Build history of the part. All positions in model axes, mm. Coordinates: 2 decimals unless noted, no trailing zeros. Order: outer loops, then holes, each group sorted by start corner. A loop starts at its lowest first (then second) coordinate and runs counter-clockwise, first axis right, second up. Notation, with made-up numbers: M -39,68 L -23,68 A18 cw -23,99 Z; hole C 1.5,65 d2. An arc over 180 degrees is marked long. Write item = value, one per line. Start each with the question number.
Q1. Band-saw the part on C-C on x = -243. Write the cut outline in (y, z).
Q2. Band-saw the part on A-A on y = -103. State how many separate pieces and enclosed holes the cut face has, plus the area to 3 significant figures.
Q3. Pin check, flat tips, straight feed: P1, Ø11.5, axis at x = -338.5, z = 202, coming from the -Y side; P2, Ø16, axis at x = 17, y = -20, coming from the +Z side; P3, Ø20, axis at x = -327, y = 292.5, coming from the +Z side. Stop position of each tip, or through.
Q4. Drill centre lines: probe 1 along Y at (x, z) = (17, 211); probe 2 along Z at (x, y) = (-330, 241.9); probe 3 along X at (y, z) = (-29, -30). Where is each one in solid material? Low to high.
Q5. Band-saw the part on B-B on z = -103. Write the cut outline in (x, y).
```python
from build123d import *

# Parameters (mm, degrees)
SKETCH1_W             = 40
SKETCH1_H             = 40
SKETCH1_W_2           = 38
SKETCH1_H_2           = 38
BOSS_EXTRUDE1_DEPTH   = 200
BOSS_EXTRUDE1_2_DEPTH = 200
BOSS_EXTRUDE1_3_DEPTH = 200
BOSS_EXTRUDE1_4_DEPTH = 200
SKETCH2_W             = 700
SKETCH2_H             = 450
SKETCH2_W_2           = 620
SKETCH2_H_2           = 370
BOSS_EXTRUDE2_DEPTH   = 40
SKETCH3_W             = 40
SKETCH3_H             = 40
SKETCH3_W_2           = 38
SKETCH3_H_2           = 38
BOSS_EXTRUDE4_DEPTH   = 100
SKETCH4_R             = 5
CUT_EXTRUDE1_DEPTH    = 465
SKETCH5_W             = 700
SKETCH5_H             = 450
SKETCH5_W_2           = 620
SKETCH5_H_2           = 370
BOSS_EXTRUDE5_DEPTH   = 40
SKETCH6_R             = 5
CUT_EXTRUDE2_DEPTH    = 508
SKETCH7_R             = 38.5
SKETCH7_R_2           = 37.5
BOSS_EXTRUDE6_DEPTH   = 5
SKETCH8_R             = 5
BOSS_EXTRUDE7_DEPTH   = 30


with BuildPart() as part:
    # Sketch1 → Boss-Extrude1 (new body, symmetric)
    with BuildSketch(Plane(origin=(0, 0, 0), x_dir=(1, 0, 0), z_dir=(0, 1, 0))):
        with Locations((-330, 205)):
            Rectangle(SKETCH1_W, SKETCH1_H)
        with Locations((-330, 205)):
            Rectangle(SKETCH1_W_2, SKETCH1_H_2, mode=Mode.SUBTRACT)
    extrude(amount=BOSS_EXTRUDE1_DEPTH, both=True)



with BuildPart() as body_2:
    # Sketch1 → Boss-Extrude1 2 (new body, symmetric)
    with BuildSketch(Plane(origin=(0, 0, 0), x_dir=(1, 0, 0), z_dir=(0, 1, 0))):
        with Locations((330, 205)):
            Rectangle(SKETCH1_W, SKETCH1_H)
        with Locations((330, 205)):
            Rectangle(SKETCH1_W_2, SKETCH1_H_2, mode=Mode.SUBTRACT)
    extrude(amount=BOSS_EXTRUDE1_2_DEPTH, both=True)


with BuildPart() as body_3:
    # Sketch1 → Boss-Extrude1 3 (new body, symmetric)
    with BuildSketch(Plane(origin=(0, 0, 0), x_dir=(1, 0, 0), z_dir=(0, 1, 0))):
        with Locations((330, -205)):
            Rectangle(SKETCH1_W, SKETCH1_H)
        with Locations((330, -205)):
            Rectangle(SKETCH1_W_2, SKETCH1_H_2, mode=Mode.SUBTRACT)
    extrude(amount=BOSS_EXTRUDE1_3_DEPTH, both=True)


with BuildPart() as body_4:
    # Sketch1 → Boss-Extrude1 4 (new body, symmetric)
    with BuildSketch(Plane(origin=(0, 0, 0), x_dir=(1, 0, 0), z_dir=(0, 1, 0))):
        with Locations((-330, -205)):
            Rectangle(SKETCH1_W, SKETCH1_H)
        with Locations((-330, -205)):
            Rectangle(SKETCH1_W_2, SKETCH1_H_2, mode=Mode.SUBTRACT)
    extrude(amount=BOSS_EXTRUDE1_4_DEPTH, both=True)


with BuildPart() as part_1:
    add(part.part)

    add(body_2.part)  # Boss-Extrude2 merges body 2

    add(body_3.part)  # Boss-Extrude2 merges body 3

    add(body_4.part)  # Boss-Extrude2 merges body 4
    # Sketch2 → Boss-Extrude2 (add)
    with BuildSketch(Plane(origin=(0, 200, 0), x_dir=(1, 0, 0), z_dir=(0, 1, 0))):
        Rectangle(SKETCH2_W, SKETCH2_H)
        Rectangle(SKETCH2_W_2, SKETCH2_H_2, mode=Mode.SUBTRACT)
    extrude(amount=BOSS_EXTRUDE2_DEPTH)

    # Sketch3 → Boss-Extrude4 (add)
    with BuildSketch(Plane(origin=(0, 240, 0), x_dir=(1, 0, 0), z_dir=(0, 1, 0))):
        with Locations((-330, 0)):
            Rectangle(SKETCH3_W, SKETCH3_H)
        with Locations((-330, 0)):
            Rectangle(SKETCH3_W_2, SKETCH3_H_2, mode=Mode.SUBTRACT)
        with Locations((330, 0)):
            Rectangle(SKETCH3_W, SKETCH3_H)
        with Locations((330, 0)):
            Rectangle(SKETCH3_W_2, SKETCH3_H_2, mode=Mode.SUBTRACT)
    extrude(amount=BOSS_EXTRUDE4_DEPTH)

    # Sketch4 → Cut-Extrude1 (cut)
    with BuildSketch(Plane.XY.offset(225)):
        with Locations((17, 220)):
            Circle(SKETCH4_R)
    extrude(amount=-CUT_EXTRUDE1_DEPTH, mode=Mode.SUBTRACT)

    # Sketch5 → Boss-Extrude5 (add)
    with BuildSketch(Plane(origin=(0, 0, 0), x_dir=(1, 0, 0), z_dir=(0, 1, 0))):
        Rectangle(SKETCH5_W, SKETCH5_H)
        Rectangle(SKETCH5_W_2, SKETCH5_H_2, mode=Mode.SUBTRACT)
    extrude(amount=-BOSS_EXTRUDE5_DEPTH)

    # Sketch6 → Cut-Extrude2 (cut)
    with BuildSketch(Plane.XY.offset(225)):
        with Locations((17, -20)):
            Circle(SKETCH6_R)
    extrude(amount=-CUT_EXTRUDE2_DEPTH, mode=Mode.SUBTRACT)

    # Sketch7 → Boss-Extrude6 (add)
    with BuildSketch(Plane(origin=(0, 240, 0), x_dir=(1, 0, 0), z_dir=(0, 1, 0))):
        with Locations((-330, 0)):
            Circle(SKETCH7_R)
        with Locations((-330, 0)):
            Circle(SKETCH7_R_2, mode=Mode.SUBTRACT)
        with Locations((330, 0)):
            Circle(SKETCH7_R)
        with Locations((330, 0)):
            Circle(SKETCH7_R_2, mode=Mode.SUBTRACT)
    extrude(amount=BOSS_EXTRUDE6_DEPTH)

    # Sketch8 → Boss-Extrude7 (add)
    with BuildSketch(Plane.XY.offset(225)):
        with Locations((-90.424393733, -20)):
            Circle(SKETCH8_R)
    extrude(amount=BOSS_EXTRUDE7_DEPTH)


solid = part_1.part
```
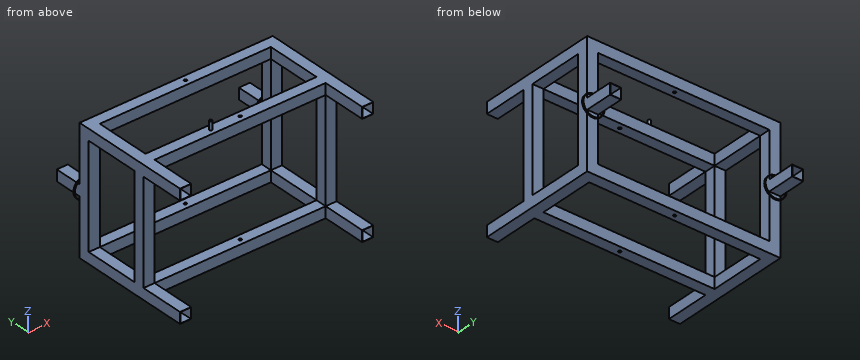
Recorded:
q1.outline = M -40,-225 L 0,-225 L 0,-185 L -40,-185 Z; M -40,185 L 0,185 L 0,225 L -40,225 Z; M 200,-225 L 240,-225 L 240,-185 L 200,-185 Z; M 200,185 L 240,185 L 240,225 L 200,225 Z
q2.separate_pieces = 4
q2.enclosed_holes = 4
q2.area = 624 mm2
q3.P1 = -40
q3.P2 = 225
q3.P3 = 20
q4.probe_1 = -40 to -25, -15 to 0, 200 to 215, 225 to 240
q4.probe_2 = -38.5 to -37.5, -20 to -19, 19 to 20, 37.5 to 38.5
q4.probe_3 = -350 to -310, 310 to 350
q5.outline = M -350,-40 L -310,-40 L -310,0 L -350,0 Z; M -350,200 L -310,200 L -310,240 L -350,240 Z; M 310,-40 L 350,-40 L 350,0 L 310,0 Z; M 310,200 L 350,200 L 350,240 L 310,240 Z
